```python
from build123d import *

# Parameters (mm, degrees)
SKETCH1_R                  = 10
BOSS_EXTRUDE1_DEPTH        = 9.525
FILLET1_R                  = 10
FILLET2_R                  = 5
M8X1_25_TAPPED_HOLE1_D     = 6.8
M8X1_25_TAPPED_HOLE1_DEPTH = 22.25
M8X1_25_TAPPED_HOLE1_TIP   = 2.042926105


with BuildPart() as part:
    # Sketch1 → Boss-Extrude1 (new body)
    with BuildSketch(Plane(origin=(0, 0, 0), x_dir=(1, 0, 0), z_dir=(0, 1, 0))):
        with BuildLine():
            Line((-7, 40), (7, 40))
            Line((7, 40), (7, 13.266499161))
            ThreePointArc((7, 13.266499161), (15, 0), (7, -13.266499161))
            Line((7, -13.266499161), (7, -23.266499161))
            Line((7, -23.266499161), (75, -47.63233641))
            Line((75, -47.63233641), (75, -75))
            ThreePointArc((75, -75), (53.765490493, -91.429054638), (29.086079144, -102))
            Line((29.086079144, -102), (-29.086079144, -102))
            ThreePointArc((-29.086079144, -102), (-53.765490493, -91.429054638), (-75, -75))
            Line((-75, -75), (-75, -47.63233641))
            Line((-75, -47.63233641), (-7, -23.266499161))
            Line((-7, -23.266499161), (-7, -13.266499161))
            ThreePointArc((-7, -13.266499161), (-15, 0), (-7, 13.266499161))
            Line((-7, 13.266499161), (-7, 40))
        make_face()
        Circle(SKETCH1_R, mode=Mode.SUBTRACT)
    extrude(amount=BOSS_EXTRUDE1_DEPTH)

    # Fillet1
    fillet1_edges = [part.edges().sort_by_distance(p)[0] for p in [
        (7, 4.7625, -13.266499161),
        (7, 4.7625, 13.266499161),
        (-7, 4.7625, 13.266499161),
        (-7, 4.7625, -13.266499161),
    ]]
    fillet(fillet1_edges, radius=FILLET1_R)

    # Fillet2
    fillet2_edges = [part.edges().sort_by_distance(p)[0] for p in [
        (7, 4.7625, 23.266499161),
        (75, 4.7625, 47.63233641),
        (75, 4.7625, 75),
        (-75, 4.7625, 75),
        (-75, 4.7625, 47.63233641),
        (-7, 4.7625, 23.266499161),
    ]]
    fillet(fillet2_edges, radius=FILLET2_R)

    # M8x1.25 Tapped Hole1
    with Locations(Plane(origin=(0, 0, -40), x_dir=(-1, 0, 0), z_dir=(0, 0, -1))):
        with Locations((0, 4.7625)):
            Hole(M8X1_25_TAPPED_HOLE1_D / 2, depth=M8X1_25_TAPPED_HOLE1_DEPTH)
            with Locations((0, 0, -(M8X1_25_TAPPED_HOLE1_DEPTH + M8X1_25_TAPPED_HOLE1_TIP / 2))):  # 118° drill point
                Cone(0, M8X1_25_TAPPED_HOLE1_D / 2, M8X1_25_TAPPED_HOLE1_TIP, mode=Mode.SUBTRACT)


solid = part.part
```
Input: part model. Units: mm. Frame: model coordinates. A direction names the side the tool comes from. Round coordinates to 2 decimals unless told otherwise and drop trailing zeros. Order: outer loops, then holes, each group sorted by start corner. A loop starts at its lowest first (then second) coordinate and runs counter-clockwise, first axis right, second up. Notation, with made-up numbers: (-11, -16) - (36, -16) arc R21 cw to (36, 12) - close; hole circle Ø5 at (-17, 50). An arc over 180 degrees is marked (long way). One line per question, with ' | ' between items. Start each with the question number.
1) Set-up query: faces 1 (the cylindrical face through (7.887, 4.829, 22.59)), 2 (the cylindrical face through (-0.443, 8.134, -28.719)), 3 (the flat face through (-7, 5, -29)), 4 (the cylindrical face through (-7.858, 4.829, 14.278)), 5 (the cylindrical face through (-74.611, 4.829, 74.834)). Return all of +Z, -Z, +X, -X, +Y, -Y with unobstructed straight access to the full face (end or side cutting, diameter ignored); none if empty.
2) Ray query, probe 1 along X at (y, z) = (7, 0); probe 2 along Z at (x, y) = (-8, 1.25); probe 3 along Y at (x, z) = (0.5, -28) (3 decimals). Return the intervals inside material, ascending.
3) Contact query for flat-ended pins moving along their axis: P1, Ø2, axis at x = -58, y = 4, coming from the -Z side; P2, Ø0.7, axis at y = 6.5, z = 19, coming from the +X side. Output: stop coordinate, or through.
4) Pull-direction query (X, two-part tool) for faces 6 (the flat face through (1, 0, 62)), 7 (the cylindrical face through (53.15, 4.7, 91.79)), 8 (the conical face through (0.077, 5.348, -16.062)), 9 (the cylindrical face through (-2.17, 4.7, 9.76)); classes: +X half, -X half, draft (parallel to the pull), parting line (faces both ways), or undercut.
5) Cut plane B-B, the plane x = -45. Return the cut outline in (y, z) (3 decimals), then the cut area to 3 significant figures.
6) Cut plane A-A, the plane z = 0. Return the cut outline in (x, y) (3 decimals), then the cut area to 4 significant figures.
7) Cut plane C-C, the plane z = 79.5. Return the cut outline in (x, y) (3 decimals), then the cut area to 3 significant figures.
Worked out:
1) face 1: +X, +Y, -Y | face 2: -Z | face 3: -Z, -X, +Y, -Y | face 4: -X, +Y, -Y | face 5: +Z, -X, +Y, -Y
2) probe 1: x = -15 to -10, 10 to 15 | probe 2: z = -13.97 to -6, 6 to 13.97, 22.75 to 102 | probe 3: y = 0 to 1.399, 8.126 to 9.525
3) P1: stops at z = 41.18 | P2: stops at x = 7
4) face 6: draft | face 7: +X half | face 8: undercut | face 9: undercut
5) outline: (0, 36.883) - (9.525, 36.883) - (9.525, 96.047) - (0, 96.047) - close | area: 564 mm^2
6) outline: (-15, 0) - (-10, 0) - (-10, 9.525) - (-15, 9.525) - close; (10, 0) - (15, 0) - (15, 9.525) - (10, 9.525) - close | area: 95.25 mm^2
7) outline: (-70.212, 0) - (70.212, 0) - (70.212, 9.525) - (-70.212, 9.525) - close | area: 1,340 mm^2
